Geometry check sheet. Reference: the model listing, model coordinates, mm. Coordinates: 2 decimals unless noted, no trailing zeros. Loops run counter-clockwise (first coordinate to the right, second up) from the corner with the lowest first, then second, coordinate; pieces in that order, holes last. Notation, with made-up numbers: (62.25, -2) - (106.25, -2) arc R30 cw to (106.25, 32) - close; hole circle Ø1 at (-16.75, 39). An arc over 180 degrees is marked (long way). Write item = value, one per line. Start each with the question number.
from build123d import *

# Parameters (mm, degrees)
BOSS_EXTRUDE1_DEPTH = 1
CUT_EXTRUDE1_REACH  = 3
SKETCH2_R           = 1


with BuildPart() as part:
    # Sketch1 → Boss-Extrude1 (new body)
    with BuildSketch(Plane(origin=(0, 0, 0), x_dir=(1, 0, 0), z_dir=(0, 1, 0))):
        Polygon((0, 0), (0, 6.4), (32.6, 6.4), (32.6, 0), (30.6, 0), (30.6, 3.2), (28.8, 3.2), (28.8, 0), (26.8, 0), (26.8, 3.2), (13.6, 3.2), (13.6, -3.6), (11.35, -3.6), (7.6, 0), (7.6, 3.2), (5.8, 3.2), (5.8, 0), (3.8, 0), (3.8, 3.2), (2, 3.2), (2, 0), align=None)
    extrude(amount=BOSS_EXTRUDE1_DEPTH)

    # Sketch2 → Cut-Extrude1 (cut, up to next)
    with BuildSketch(Plane(origin=(0, 1, 0), x_dir=(1, 0, 0), z_dir=(0, 1, 0)), mode=Mode.PRIVATE) as cut_extrude1_sk1:
        with Locations((9.286488836, 4.615010183)):
            Circle(SKETCH2_R)
    cut_extrude1_tool1 = extrude(cut_extrude1_sk1.sketch, amount=-CUT_EXTRUDE1_REACH, mode=Mode.PRIVATE) & part.part
    add(cut_extrude1_tool1.solids().sort_by_distance((9.286489, 1, -4.61501))[0], mode=Mode.SUBTRACT)
    # Sketch2 → Cut-Extrude1 (cut, up to next)
    with BuildSketch(Plane(origin=(0, 1, 0), x_dir=(1, 0, 0), z_dir=(0, 1, 0)), mode=Mode.PRIVATE) as cut_extrude1_sk2:
        with Locations((12.147825288, 1.964747252)):
            Circle(SKETCH2_R)
    cut_extrude1_tool2 = extrude(cut_extrude1_sk2.sketch, amount=-CUT_EXTRUDE1_REACH, mode=Mode.PRIVATE) & part.part
    add(cut_extrude1_tool2.solids().sort_by_distance((12.147825, 1, -1.964747))[0], mode=Mode.SUBTRACT)
    # Sketch2 → Cut-Extrude1 (cut, up to next)
    with BuildSketch(Plane(origin=(0, 1, 0), x_dir=(1, 0, 0), z_dir=(0, 1, 0)), mode=Mode.PRIVATE) as cut_extrude1_sk3:
        with Locations((12.147825288, -1.494058873)):
            Circle(SKETCH2_R)
    cut_extrude1_tool3 = extrude(cut_extrude1_sk3.sketch, amount=-CUT_EXTRUDE1_REACH, mode=Mode.PRIVATE) & part.part
    add(cut_extrude1_tool3.solids().sort_by_distance((12.147825, 1, 1.494059))[0], mode=Mode.SUBTRACT)


solid = part.part
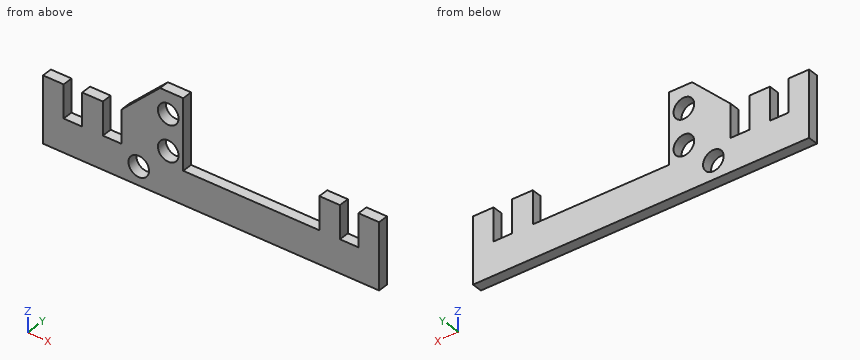
(1) Sectioned sample at B-B on x = 10. Enter the section's corners in (y, z), plus the area to 3 significant figures.
(2) Scan lines: line 1 (X direction, y = 0.2, z = -0.75); line 2 (Z direction, x = 13, y = 0.4); line 3 (Z direction, x = 3, y = 0.55). Record each from-to range of solid material in increasing order.
(3) Sectioned sample at C-C on z = 1. Enter the section's corners in (x, y).
(4) Depth check by flat-ended pin: pin 1 (0.5 mm diameter, centred on x = 5, y = 0.5, fed in from +Z). Enter the tip coordinate at first touch or a pass-through.
(5) Sectioned sample at A-A on z = -0.5. Enter the section's corners in (x, y).
(6) Sectioned sample at D-D on y = 0.8. Enter the section's corners in (x, z).
Working result:
q1.outline = (0, -6.4) - (1, -6.4) - (1, -5.32) - (0, -5.32) - close; (0, -3.91) - (1, -3.91) - (1, 2.3) - (0, 2.3) - close
q1.area = 7.30 mm2
q2.line_1 = 0 to 2, 3.8 to 5.8, 7.6 to 13.6, 26.8 to 28.8, 30.6 to 32.6
q2.line_2 = -6.4 to -2.49, -1.44 to 0.97, 2.02 to 3.6
q2.line_3 = -6.4 to -3.2
q3.outline = (8.64, 0) - (11.28, 0) - (11.28, 1) - (8.64, 1) - close; (13.02, 0) - (13.6, 0) - (13.6, 1) - (13.02, 1) - close
q4.pin_1 = 0
q5.outline = (0, 0) - (2, 0) - (2, 1) - (0, 1) - close; (3.8, 0) - (5.8, 0) - (5.8, 1) - (3.8, 1) - close; (7.6, 0) - (13.6, 0) - (13.6, 1) - (7.6, 1) - close; (26.8, 0) - (28.8, 0) - (28.8, 1) - (26.8, 1) - close; (30.6, 0) - (32.6, 0) - (32.6, 1) - (30.6, 1) - close
q6.outline = (0, -6.4) - (32.6, -6.4) - (32.6, 0) - (30.6, 0) - (30.6, -3.2) - (28.8, -3.2) - (28.8, 0) - (26.8, 0) - (26.8, -3.2) - (13.6, -3.2) - (13.6, 3.6) - (11.35, 3.6) - (7.6, 0) - (7.6, -3.2) - (5.8, -3.2) - (5.8, 0) - (3.8, 0) - (3.8, -3.2) - (2, -3.2) - (2, 0) - (0, 0) - close; hole circle Ø2 at (9.29, -4.62); hole circle Ø2 at (12.15, -1.96); hole circle Ø2 at (12.15, 1.49)
